Autodesk Inventor part; units mm, degrees
ref_plane "YZ Plane" through (0, 0, 0) normal (1, 0, 0) x (0, 1, 0)
ref_plane "XZ Plane" through (0, 0, 0) normal (0, 1, 0) x (-1, 0, 0)
ref_plane "XY Plane" through (0, 0, 0) normal (0, 0, 1) x (1, 0, 0)
sketch "草图1" plane through (0, 0, 0) normal (0, 0, 1) x (1, 0, 0)
  circle A0 centre (0, 0) radius 20
  dimension "d0" = 40
extrude "拉伸1" add sketch "草图1" along normal blind 160
sketch "草图2" plane through (0, 0, 160) normal (0, 0, 1) x (1, 0, 0)
  line L0 (-40, 0) -> (40, 0)
  line L1 (40, 0) -> (40, -30) construction
  line L2 (40, -30) -> (-40, -30)
  line L3 (-40, -30) -> (-40, 0) construction
  circle A0 centre (0, 0) radius 20
  line L4 (-20, 80) -> (20, 80)
  line L5 (20, 80) -> (20, -30)
  line L6 (20, -30) -> (-20, -30)
  line L7 (-20, -30) -> (-20, 80)
  line L8 (-20, 80) -> (-40, -30)
  line L9 (0, 0) -> (0, 63.2823)
  line L10 (20, 80) -> (40, -30)
  arc A1 (-20, 80) -> (-40, -30) centre (199.6341, -16.7516) ccw
  arc A2 (40, -30) -> (20, 80) centre (-199.6341, -16.7516) ccw
  arc A3 (20, 80) -> (-20, 80) centre (0, 45.359) ccw
  circle A4 centre (0, 120.4047) radius 25
  circle A5 centre (0, 0) radius 75
  line L11 (2.3516, 185.7586) -> (-119.2479, -80.6225)
  point P0 (0, -30)
  dimension "d3" = 80
  dimension "d4" = 30
  dimension "d5" = 40
  dimension "d6" = 110
  dimension "d7" = 20
  dimension "d8" = 110
  dimension "d9" = 240
  dimension "d10" = 40
  dimension "d24" = 50
  dimension "d25" = 150
extrude "拉伸2" add sketch "草图2" along normal blind 15 contours L9 A0 L0 | L0 A0 | L0 A0 L9 | L5 A5 L10 L0 | L5 L2 L7 A0 | L0 L10 L2 L5 | A0 L7 A5 L5 | L7 L2 L8 L0 | L0 L8 A5 L7 | L10 A5 A2 L0 | L0 A2 L10 | A5 L7 L4 L5 | L5 L10 A5 | L8 A1 L0 | L0 A1 A5 L8 | A5 L8 L7 | L10 A2 A5 | L4 A3 | A5 A1 L8
sketch "草图3" plane through (0, 0, 175) normal (0, 0, 1) x (1, 0, 0)
  circle A0 centre (0, 60) radius 20
  point P0 (0, 0)
  dimension "d13" = 40
  dimension "d14" = 60
extrude "拉伸3" add sketch "草图3" along normal blind 80
ref_plane "工作平面1" through (0, 60, 215) normal (0, 0, 1) x (1, 0, 0)
mirror "镜像1" about plane through (0, 60, 215) normal (0, 0, 1) of "拉伸2"
mirror "镜像2" about plane through (0, 60, 215) normal (0, 0, 1) of "拉伸1"
sketch "草图4" plane through (0, 0, 430) normal (0, 0, 1) x (1, 0, 0)
  circle A0 centre (0, 0) radius 20
hole "孔1" at (0, 0, 430) direction (0, 0, -1) diameter 30 depth 40
mirror "镜像3" about plane through (0, 60, 215) normal (0, 0, 1) of "孔1"
equation "\"d8\" = 5.5 * d7"
properties part number "曲轴"
CAD build for the part. Positions are in the model's coordinates, mm. A direction names the side the tool comes from. Round coordinates to 2 decimals unless told otherwise and drop trailing zeros. Order: outer loops, then holes, each group sorted by start corner. A loop starts at its lowest first (then second) coordinate and runs counter-clockwise, first axis right, second up.
Q1. Which spindle directions (+Z, -Z, +X, -X, +Y, -Y) get a long thin tool onto all of the face, cutting with end or side? Do faces 1 (the cylindrical face through (-4.336, -19.524, 351.12)), 2 (the cylindrical face through (0.66, 14.985, 20.28)), 3 (the cylindrical face through (-4.336, 79.524, 214.44)). Say none if no direction does.
Q2. Slice it at B-B (x = 0). Write the cut outline in (y, z).
Q3. Slice it at A-A (x = 26). Write the cut outline in (y, z), and give its area (3 significant figures).
Q4. Drop flat-ended pins along their axis: pin 1 (5 mm diameter, centred on x = 25.5, y = -2, fed in from -Z); pin 2 (1 mm diameter, centred on x = 8.5, z = 340, fed in from -Y); pin 3 (1.5 mm diameter, centred on x = 13, z = 218, fed in from +Y). Give the stop position or say it passes through.
Q5. Wall check: L1, parallel to Y at x = 0, z = 421; L2, parallel to Z at x = 26.5, y = 4.5; L3, parallel to Z at x = -16, y = -8. Give the ranges that are in metal, low to high.
Q6. Two-plate mould, pull along Y, no slides. Class faces 4 (the flat face through (-1, -30, 263)), 5 (the cylindrical face through (-0.66, 14.985, 409.72)), 6 (the flat face through (-3, 15, 430)): pulls with the +Y half, pulls with the -Y half, needs draft (parallel to the pull), parting line crosses it, or undercut.
Q7. Slice it at D-D (z = 28). Write the cut outline in (x, y).
Q8. Slice it at C-C (y = 0). Write the cut outline in (x, z).
Results below:
1. face 1: +Z
1. face 2: -Z
1. face 3: none
2. outline: (-30, 160) - (-20, 160) - (-20, 0) - (-15, 0) - (-15, 40) - (15, 40) - (15, 0) - (20, 0) - (20, 160) - (85.36, 160) - (85.36, 175) - (80, 175) - (80, 255) - (85.36, 255) - (85.36, 270) - (20, 270) - (20, 430) - (15, 430) - (15, 390) - (-15, 390) - (-15, 430) - (-20, 430) - (-20, 270) - (-30, 270) - (-30, 255) - (40, 255) - (40, 175) - (-30, 175) - close
3. outline: (-30, 160) - (65.04, 160) - (65.04, 175) - (-30, 175) - close; (-30, 255) - (65.04, 255) - (65.04, 270) - (-30, 270) - close
3. area: 2,850 mm2
4. pin 1: stops at z = 160
4. pin 2: stops at y = -18.33
4. pin 3: stops at y = 75.81
5. L1: y = -20 to -15, 15 to 20
5. L2: z = 160 to 175, 255 to 270
5. L3: z = 0 to 175, 255 to 430
6. face 4: pulls with the -Y half
6. face 5: undercut
6. face 6: needs draft
7. outline: circle Ø40 at (0, 0); hole circle Ø30 at (0, 0)
8. outline: (-39.78, 160) - (-20, 160) - (-20, 0) - (-15, 0) - (-15, 40) - (15, 40) - (15, 0) - (20, 0) - (20, 160) - (39.78, 160) - (39.78, 175) - (-39.78, 175) - close; (-39.78, 255) - (39.78, 255) - (39.78, 270) - (20, 270) - (20, 430) - (15, 430) - (15, 390) - (-15, 390) - (-15, 430) - (-20, 430) - (-20, 270) - (-39.78, 270) - close
